Build history of the part. All positions in model axes, mm. Face numbers are marked on the shaded views. A direction names the side the tool comes from. Round coordinates to 2 decimals unless told otherwise and drop trailing zeros. Write each loop counter-clockwise with the first axis right and the second up, starting at its lowest first coordinate (ties: lowest second). Pieces come first, ordered by that corner, then holes. Notation, with made-up numbers: M 52.5,-8 L 102.5,-8 A18 cw 102.5,10 Z; hole C -33,48 d5. An arc over 180 degrees is marked long. Write item = value, one per line. Start each with the question number.
Q1. Tool access for the marked faces 1 and 2: list every direction of +Z, -Z, +X, -X, +Y, -Y with a clear straight run to the whole face (end or side of a thin tool).
Q2. Band-saw the part on A-A on y = 6.25. Write the cut outline in (x, z).
Q3. Probe L1, parallel to X at y = 9.75, z = 7.5; L2, parallel to Z at x = 8.75, y = 1; L3, parallel to Z at x = 7.5, y = 2.25. List the from-to ranges inside material, lowest first.
Q4. Band-saw the part on C-C on y = 14. Write the cut outline in (x, z), plus the area to 3 significant figures.
Q5. Pull direction Y, two halves, no side cores. Call the marked faces 3, 4, 5 and 6: released by +Y, released by -Y, zero draft, split by the parting line, or undercut.
Q6. Drop flat-ended pins along their axis: P1, Ø1, axis at x = 2.5, y = 14, coming from the +Z side; P2, Ø8, axis at x = 9, z = 4.5, coming from the -Y side; P3, Ø5, axis at x = 5.5, z = 5, coming from the +Y side. Give the stop position or say it passes through.
Q7. Band-saw the part on B-B on y = 1.25. Write the cut outline in (x, z), plus the area to 3 significant figures.
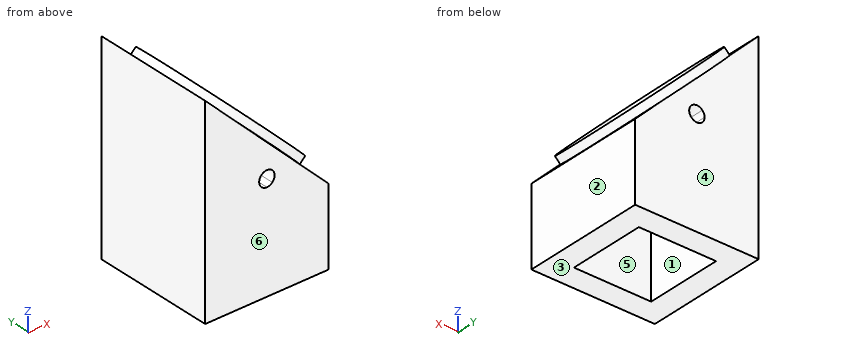
```python
from build123d import *

# Parameters (mm, degrees)
SKETCH_1_W          = 16
SKETCH_1_H          = 16
SKETCH_1_W_2        = 10
SKETCH_1_H_2        = 10
EXTRUDE_1_DEPTH     = 10
EXTRUDE_2_DEPTH     = 16
EXTRUDE_3_DEPTH     = 1
CUT_EXTRUDE_3_DEPTH = 16


with BuildPart() as part:
    # 草图1 → 凸台-拉伸1 (new body)
    with BuildSketch(Plane.XY):
        with Locations((8, 8)):
            Rectangle(SKETCH_1_W, SKETCH_1_H)
        with Locations((8, 8)):
            Rectangle(SKETCH_1_W_2, SKETCH_1_H_2, mode=Mode.SUBTRACT)
    extrude(amount=EXTRUDE_1_DEPTH)

    # 草图2 → 凸台-拉伸2 (add)
    with BuildSketch(Plane.XZ):
        Polygon((0, 10), (0, 26), (16, 10), align=None)
    extrude(amount=-EXTRUDE_2_DEPTH)

    # 草图6 → 凸台-拉伸3 (add)
    with BuildSketch(Plane(origin=(13, 0, 13), x_dir=(0.7071067811865475, 0, -0.7071067811865477), z_dir=(0.7071067811865477, 0, 0.7071067811865475))):
        with BuildLine():
            Line((-13.071067812, 0), (-7.071067812, 0))
            Line((-7.071067812, 0), (-7.071067812, 16))
            Line((-7.071067812, 16), (-13.071067812, 16))
            ThreePointArc((-13.071067812, 16), (-17.071067812, 8), (-13.071067812, 0))
        make_face()
        with BuildLine():
            Line((-7.071067812, 16), (-7.071067812, 0))
            Line((-7.071067812, 0), (-1.071067812, 0))
            ThreePointArc((-1.071067812, 0), (1.873204098, 3.527864045), (2.928932188, 8))
            ThreePointArc((2.928932188, 8), (1.873204098, 12.472135955), (-1.071067812, 16))
            Line((-1.071067812, 16), (-7.071067812, 16))
        make_face()
        with BuildLine():
            Line((-1.071067812, 0), (-7.071067812, 0))
            Line((-7.071067812, 0), (-13.071067812, 0))
            ThreePointArc((-13.071067812, 0), (-7.071067812, -2), (-1.071067812, 0))
        make_face()
        with BuildLine():
            Line((-13.071067812, 16), (-7.071067812, 16))
            Line((-7.071067812, 16), (-1.071067812, 16))
            ThreePointArc((-1.071067812, 16), (-7.071067812, 18), (-13.071067812, 16))
        make_face()
    extrude(amount=EXTRUDE_3_DEPTH)

    # 草图9 → 切除-拉伸3 (cut)
    with BuildSketch(Plane(origin=(0, 0, 0), x_dir=(-1, 0, 0), z_dir=(0, -1, 0))):
        with BuildLine():
            Line((-8, -13.757359313), (-7.292893219, -14.464466094))
            ThreePointArc((-7.292893219, -14.464466094), (-7.076120467, -14.140042745), (-7, -13.757359313))
            ThreePointArc((-7, -13.757359313), (-7.292893219, -13.050252532), (-8, -12.757359313))
            Line((-8, -12.757359313), (-8, -13.757359313))
        make_face()
        with BuildLine():
            Line((-8.707106781, -13.050252532), (-8, -13.757359313))
            Line((-8, -13.757359313), (-8, -12.757359313))
            ThreePointArc((-8, -12.757359313), (-8.382683432, -12.83347978), (-8.707106781, -13.050252532))
        make_face()
        with BuildLine():
            ThreePointArc((-8.707106781, -13.050252532), (-8.707106781, -14.464466094), (-7.292893219, -14.464466094))
            Line((-7.292893219, -14.464466094), (-8, -13.757359313))
            Line((-8, -13.757359313), (-8.707106781, -13.050252532))
        make_face()
    extrude(amount=-CUT_EXTRUDE_3_DEPTH, mode=Mode.SUBTRACT)


solid = part.part
```
Conclusion:
q1.face_1 = -Z
q1.face_2 = +Z, -Z, +X, +Y, -Y
q2.outline = M 0,0 L 3,0 L 3,10 L 13,10 L 13,0 L 16,0 L 16,10 L 14.96,11.04 L 15.67,11.75 L 1.75,25.67 L 1.04,24.96 L 0,26 Z; hole C 8,13.76 d2
q3.L1 = 0 to 3, 13 to 16
q3.L2 = 0 to 13.1, 14.42 to 18.66
q3.L3 = 0 to 12.89, 14.62 to 19.91
q4.outline = M 0,0 L 16,0 L 16,10 L 13.66,12.34 L 14.36,13.05 L 3.05,24.36 L 2.34,23.66 L 0,26 Z; hole C 8,13.76 d2
q4.area = 301 mm^2
q5.face_3 = zero draft
q5.face_4 = released by +Y
q5.face_5 = undercut
q5.face_6 = released by -Y
q6.P1 = 24.53
q6.P2 = 0
q6.P3 = 16
q7.outline = M 0,0 L 16,0 L 16,10 L 13.22,12.78 L 13.92,13.49 L 3.49,23.92 L 2.78,23.22 L 0,26 Z; hole C 8,13.76 d2
q7.area = 300 mm^2
